Read the model definition and answer for the solid it produces. Units are mm, in the model's axes. Face numbers are marked on the shaded views. A direction names the side the tool comes from. Coordinates: 2 decimals unless noted, no trailing zeros. Write each loop counter-clockwise with the first axis right and the second up, starting at its lowest first coordinate (ties: lowest second). Pieces come first, ordered by that corner, then holes.
(1) Given pin 1 (1 mm diameter, centred on x = -0.5, z = 1, fed in from +Y); pin 2 (3 mm diameter, centred on x = 4, z = 2, fed in from -Y), each flat-ended and moving along its own axis, determine where each tip first touches the part or whether it passes through.
(2) The part is cut by section C-C, the plane z = -1.7. Determine the outline of the cut face in (x, y), and give its area (3 significant figures).
(3) The part is cut by section D-D, the plane x = 4. Determine the outline of the cut face in (y, z).
(4) Straight lines are drawn through the part: line 1 along Z through (x, y) = (-1, -0.05); line 2 along X through (y, z) = (0, 0.35); line 3 along Y through (x, z) = (6.25, 0.5). For each, find the intervals that lie inside material, in ascending order.
(5) The part is cut by section B-B, the plane x = 0. Determine the outline of the cut face in (y, z).
(6) Which of the six approach directions +Z, -Z, +X, -X, +Y, -Y give full straight-line access (tool end or side, diameter ignored) to the marked faces 1, 2, 3 and 4?
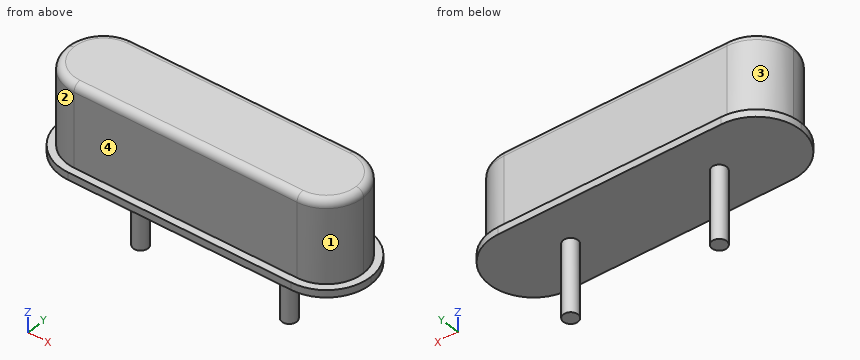
```python
from build123d import *

# Parameters (mm, degrees)
SKETCH2_R           = 0.254
SKETCH4_W           = 10.16
SKETCH4_H           = 3.093614779
BOSS_EXTRUDE1_DEPTH = 1.27
FILLET1_R           = 1.27
FILLET2_R           = 0.254
BOSS_EXTRUDE2_DEPTH = 0.254


with BuildPart() as part:
    # Base-Sweep: sweep along a path in Sketch1
    with BuildLine(Plane(origin=(0, 0, 0), x_dir=(1, 0, 0), z_dir=(0, 1, 0))) as base_sweep_path:
        Line((0, 2.54), (0, -0.508))
    # Sketch2 → Base-Sweep (sweep)
    with BuildSketch(Plane.XY.offset(-2.54)):
        Circle(SKETCH2_R)
    base_sweep = sweep(path=base_sweep_path.line)

    # Sketch4 → Boss-Extrude1 (add, symmetric)
    with BuildSketch(Plane(origin=(0, 0, 0), x_dir=(1, 0, 0), z_dir=(0, 1, 0))):
        with Locations((2.54, -1.54680739)):
            Rectangle(SKETCH4_W, SKETCH4_H)
    extrude(amount=BOSS_EXTRUDE1_DEPTH, both=True)

    # Fillet1
    fillet1_edges = [part.edges().sort_by_distance(p)[0] for p in [
        (-2.54, -1.27, 1.546807389),
        (7.62, -1.27, 1.546807389),
        (-2.54, 1.27, 1.546807389),
        (7.62, 1.27, 1.546807389),
    ]]
    fillet(fillet1_edges, radius=FILLET1_R - 0.0001)  # a hair under: the kernel refuses the full size

    # Fillet2
    fillet2_edges = [part.edges().sort_by_distance(p)[0] for p in [
        (2.54, -1.27, 3.093614779),
        (2.54, 1.27, 3.093614779),
        (7.248054901, 0.898054901, 3.093614779),
        (7.248054901, -0.898054901, 3.093614779),
        (-2.168054901, 0.898054901, 3.093614779),
        (-2.168054901, -0.898054901, 3.093614779),
    ]]
    fillet(fillet2_edges, radius=FILLET2_R)

    # Mirror5: Base-Sweep across plane
    add(base_sweep.mirror(Plane(origin=(2.54, 0, 0), x_dir=(0, 0, 1), z_dir=(1, 0, 0))))

    # Sketch6 → Boss-Extrude2 (add)
    with BuildSketch(Plane(origin=(0, 0, 0), x_dir=(-1, 0, 0), z_dir=(0, 0, -1))):
        with BuildLine():
            Line((-6.35, -1.524), (1.27, -1.524))
            ThreePointArc((1.27, -1.524), (2.347630735, -1.077630735), (2.794, 0))
            ThreePointArc((2.794, 0), (2.347630735, 1.077630735), (1.27, 1.524))
            Line((1.27, 1.524), (-6.35, 1.524))
            ThreePointArc((-6.35, 1.524), (-7.427630735, 1.077630735), (-7.874, 0))
            ThreePointArc((-7.874, 0), (-7.427630735, -1.077630735), (-6.35, -1.524))
        make_face()
    extrude(amount=-BOSS_EXTRUDE2_DEPTH)


solid = part.part
```
Computed:
1. pin 1: stops at y = 1.27
1. pin 2: stops at y = -1.27
2. outline: circle Ø0.51 at (0, 0); circle Ø0.51 at (5.08, 0)
2. area: 0.405 mm2
3. outline: (-1.52, 0) - (1.52, 0) - (1.52, 0.25) - (1.27, 0.25) - (1.27, 2.84) arc R0.25 ccw to (1.02, 3.09) - (-1.02, 3.09) arc R0.25 ccw to (-1.27, 2.84) - (-1.27, 0.25) - (-1.52, 0.25) - close
4. line 1: z = 0 to 3.09
4. line 2: x = -2.54 to 7.62
4. line 3: y = -1.27 to 1.27
5. outline: (-1.52, 0) - (-0.25, 0) - (-0.25, -2.54) - (0.25, -2.54) - (0.25, 0) - (1.52, 0) - (1.52, 0.25) - (1.27, 0.25) - (1.27, 2.84) arc R0.25 ccw to (1.02, 3.09) - (-1.02, 3.09) arc R0.25 ccw to (-1.27, 2.84) - (-1.27, 0.25) - (-1.52, 0.25) - close
6. face 1: +Z, +X, -Y
6. face 2: +Z, -X, -Y
6. face 3: +Z, -X, +Y
6. face 4: +Z, +X, -X, -Y
